from build123d import *
from OCP.BRepFilletAPI import BRepFilletAPI_MakeChamfer

# Parameters (mm, degrees)
BOSS_EXTRU_1_DEPTH      = 15
CHANFREIN1_SIZE         = 15
CHANFREIN1_SIZE_2       = 10.503113073
ESQUISSE4_R             = 2
ENL_V_MAT_EXTRU_3_DEPTH = 4
ENL_V_MAT_EXTRU_5_DEPTH = 5
ESQUISSE6_R             = 2
ENL_V_MAT_EXTRU_6_DEPTH = 5


with BuildPart() as part:
    # Esquisse1 → Boss.-Extru.1 (new body)
    with BuildSketch(Plane(origin=(0, 0, 0), x_dir=(1, 0, 0), z_dir=(0, 1, 0))):
        Polygon((-41.352348911, -18.647651089), (8.647651089, -18.647651089), (8.647651089, -68.647651089), (68.647651089, -68.647651089), (68.647651089, -46.647651089), (30.647651089, -46.647651089), (30.647651089, 3.352348911), (-19.352348911, 3.352348911), (-19.352348911, 41.352348911), (-41.352348911, 41.352348911), align=None)
    extrude(amount=BOSS_EXTRU_1_DEPTH)

    # Chanfrein1
    chanfrein1_edges_1 = [part.edges().sort_by_distance(p)[0] for p in [
        (38.647651089, 15, 68.647651089),
    ]]
    chanfrein1_side_1 = [part.faces().sort_by_distance(p)[0] for p in [
        (38.647651089, 14.789937739, 68.647651089),
    ]]
    chanfrein1_edges_2 = [part.edges().sort_by_distance(p)[0] for p in [
        (8.647651089, 15, 43.647651089),
    ]]
    chanfrein1_side_2 = [part.faces().sort_by_distance(p)[0] for p in [
        (8.647651089, 14.789937739, 43.647651089),
    ]]
    chanfrein1_edges_3 = [part.edges().sort_by_distance(p)[0] for p in [
        (-16.352348911, 15, 18.647651089),
    ]]
    chanfrein1_side_3 = [part.faces().sort_by_distance(p)[0] for p in [
        (-16.352348911, 14.789937739, 18.647651089),
    ]]
    chanfrein1_edges_4 = [part.edges().sort_by_distance(p)[0] for p in [
        (-41.352348911, 15, -11.352348911),
    ]]
    chanfrein1_side_4 = [part.faces().sort_by_distance(p)[0] for p in [
        (-41.352348911, 14.789937739, -11.352348911),
    ]]
    chanfrein1 = BRepFilletAPI_MakeChamfer(part.part.solid().wrapped)
    for e in chanfrein1_edges_1:
        chanfrein1.Add(CHANFREIN1_SIZE - 0.0001, CHANFREIN1_SIZE_2 - 0.0001, e.wrapped, chanfrein1_side_1[0].wrapped)
    for e in chanfrein1_edges_2:
        chanfrein1.Add(CHANFREIN1_SIZE - 0.0001, CHANFREIN1_SIZE_2 - 0.0001, e.wrapped, chanfrein1_side_2[0].wrapped)
    for e in chanfrein1_edges_3:
        chanfrein1.Add(CHANFREIN1_SIZE - 0.0001, CHANFREIN1_SIZE_2 - 0.0001, e.wrapped, chanfrein1_side_3[0].wrapped)
    for e in chanfrein1_edges_4:
        chanfrein1.Add(CHANFREIN1_SIZE - 0.0001, CHANFREIN1_SIZE_2 - 0.0001, e.wrapped, chanfrein1_side_4[0].wrapped)
    add(Compound.cast(chanfrein1.Shape()), mode=Mode.REPLACE)  # a hair under: the kernel refuses the full size

    # Esquisse4 → Enlèv. mat.-Extru.3 (cut)
    with BuildSketch(Plane.XZ):
        with Locations(Location((38.647651089, 63.647651089, 0), (0, 0, 270))):
            Circle(ESQUISSE4_R)
        with Locations(Location((13.647651089, 38.647651089, 0), (0, 0, 270))):
            Circle(ESQUISSE4_R)
        with Locations(Location((-11.352348911, 13.647651089, 0), (0, 0, 270))):
            Circle(ESQUISSE4_R)
    extrude(amount=-ENL_V_MAT_EXTRU_3_DEPTH, mode=Mode.SUBTRACT)

    # Esquisse5 → Enlèv. mat.-Extru.5 (cut)
    with BuildSketch(Plane(origin=(0, 15, 0), x_dir=(1, 0, 0), z_dir=(0, 1, 0))):
        Polygon((-28.849235838, 41.352348911), (-19.352348911, 41.352348911), (-19.352348911, 3.352348911), (30.647651089, 3.352348911), (30.647651089, -46.647651089), (68.647651089, -46.647651089), (68.647651089, -56.140382231), (21.150764162, -56.140382231), (21.150764162, -6.144538016), (-28.849235838, -6.144538016), align=None)
    extrude(amount=-ENL_V_MAT_EXTRU_5_DEPTH, mode=Mode.SUBTRACT)

    # Esquisse6 → Enlèv. mat.-Extru.6 (cut)
    with BuildSketch(Plane(origin=(0, 10, 0), x_dir=(1, 0, 0), z_dir=(0, 1, 0))):
        with Locations(Location((-23.849235838, 18.855461984, 0), (0, 0, 270))):
            Circle(ESQUISSE6_R)
        with Locations(Location((26.150764162, -1.144538016, 0), (0, 0, 270))):
            Circle(ESQUISSE6_R)
        with Locations(Location((46.150764162, -51.140382231, 0), (0, 0, 270))):
            Circle(ESQUISSE6_R)
    extrude(amount=-ENL_V_MAT_EXTRU_6_DEPTH, mode=Mode.SUBTRACT)


solid = part.part
Design review of the part built by this model. Coordinates are the model's own, in mm. A direction names the side the tool comes from. Give positions to 0.01 mm unless a question says otherwise; leave off trailing zeros. Loops run counter-clockwise (first coordinate to the right, second up) from the corner with the lowest first, then second, coordinate; pieces in that order, holes last. Notation, with made-up numbers: M 48,-6.5 L 71,-6.5 A25 ccw 71,18.5 Z; hole C 69.25,-4.5 d11. An arc over 180 degrees is marked long. Write item = value, one per line.
Q1. Insertion check: pin 1 (3 mm diameter, centred on x = 53.5, y = 5, fed in from -Z); pin 2 (8 mm diameter, centred on y = 3.5, z = 1.5, fed in from +X); pin 3 (1.5 mm diameter, centred on x = -13.5, y = 13, fed in from -Z). Each pin has a flat end and moves straight along its axis. Give the tip position at first contact, or say it passes through.
Output values:
pin_1 = 46.65
pin_2 = 30.65
pin_3 = 6.14
Q2. Draft analysis for pull direction Z (two halves, no side actions). For faces 5 (the flat face through (46, 5, 51)), 6 (the flat face through (-11.52, 7.61, 13.32)), 7 (the flat face through (-19.352, 5, -22)), state which applies: +Z half, -Z half, draft (parallel to the pull), parting line (faces both ways), or undercut.
Output values:
face_5 = undercut
face_6 = +Z half
face_7 = draft
Q3. To check wall thickness, follow line 1 (Y direction, x = 17, z = 6); line 2 (Z direction, x = -20, y = 14.25); line 3 (Z direction, x = 44, y = 11.75). State the ranges of each line that lie inside material, in increasing order. Write a range as [from, to].
Output values:
line_1 = [0, 10]
line_2 = [6.14, 8.67]
line_3 = [56.14, 60.42]
Q4. We need section B-B (y = 7). Give the boundary of the cut face in (x, z).
Output values:
outline = M -36.45,-41.35 L -19.35,-41.35 L -19.35,-3.35 L 30.65,-3.35 L 30.65,46.65 L 68.65,46.65 L 68.65,63.75 L 13.55,63.75 L 13.55,13.75 L -36.45,13.75 Z; hole C -23.85,-18.86 d4; hole C 26.15,1.14 d4; hole C 46.15,51.14 d4
Q5. For faces 1 (the flat face through (-3, 13, 6.145)), 2 (the flat face through (-24, 5, -19)), 3 (the flat face through (50, 5, 46.648)), 4 (the cylindrical face through (11.7, 2, 39.1)), list the 3-axis set-ups (+Z, -Z, +X, -X, +Y, -Y) from which the entire face can be reached by the end or side of a thin tool; tool diameter is ignored.
Output values:
face_1 = -Z, +X, +Y
face_2 = +Y
face_3 = -Z, +X, +Y, -Y
face_4 = -Y
